CAD build for the part. Positions are in the model's coordinates, mm. A direction names the side the tool comes from. Round coordinates to 2 decimals unless told otherwise and drop trailing zeros. Write each loop counter-clockwise with the first axis right and the second up, starting at its lowest first coordinate (ties: lowest second). Pieces come first, ordered by that corner, then holes. Notation, with made-up numbers: (10, 32) -> (47, 32) arc R22 ccw to (47, 39) -> close; hole circle Ø8 at (80, 18.5). An arc over 180 degrees is marked (long way). Put each result on its own line as item: value. Start each with the question number.
1. Saw through at D-D on y = -9.25. List the corners of the cut face in (x, z), and give its area (3 significant figures).
2. Pull direction X, two halves, no side cores. Call faces 4 (the cylindrical face through (-7.908, -2.465, 5.805)), 5 (the flat face through (7, -5, -7)), 6 (the flat face through (0, -15, 0)), 7 (the cylindrical face through (-0.867, 0.296, -3.905)): pulls with the +X half, pulls with the -X half, needs draft (parallel to the pull), parting line crosses it, or undercut.
3. 3-axis set-ups, long thin cutter, end or side, ignore diameter. For faces 1 (the flat face through (-4, -10, 4)), 2 (the cylindrical face through (9.139, -7.395, 14.334)), 3 (the flat face through (6, -5, 6)): which of +Z, -Z, +X, -X, +Y, -Y reach the whole face in a straight line?
4. Saw through at B-B on x = 0. List the corners of the cut face in (y, z) (3 decimals).
5. Flat gauge pins, fed straight in: P1, Ø3, axis at x = -1.5, z = -5, coming from the +Y side; P2, Ø2.5, axis at x = 5.66, z = 5.66, coming from the +Y side; P3, Ø3, axis at y = -9.5, z = 6, coming from the -X side. Where does each tip first touch, or does it go through?
6. Saw through at A-A on y = -13. List the corners of the cut face in (x, z).
7. Saw through at C-C on z = 0. List the corners of the cut face in (x, y) (3 decimals), and give its area (3 significant figures).
8. Drill centre lines: line 1 (Z direction, x = -6, y = -4.5); line 2 (Y direction, x = -0.5, z = -6.5); line 3 (Y direction, x = 2, z = -3). Where is each one in solid material? Low to high. Write a range as from..to.
from build123d import *

# Parameters (mm, degrees)
F0_R     = 17
F0_R_2   = 1.5
F0_R_3   = 1
F0_R_4   = 4
F0_R_5   = 1.475
F1_DEPTH = 15
F2_START = 10
F2_DEPTH = 15
F3_DEPTH = 5
F4_DEPTH = 0.6
F5_DEPTH = 1.2


# Not quite as in the source:
# - a feature names something its author has since deleted; it is built from what else it names


with BuildPart() as f1:
    # F0 (on Front) → F1 (new body)
    with BuildSketch(Plane.XZ):
        Circle(F0_R)
        with BuildLine():
            ThreePointArc((-4.2152867015, -5.2422664968), (-4.1715341961, -5.447511614), (-4.1568542495, -5.6568542495))
            ThreePointArc((-4.1568542495, -5.6568542495), (-6.8551617286, -6.5591065343), (-5.2422664968, -4.2152867015))
            ThreePointArc((-5.2422664968, -4.2152867015), (-4.2289624147, -3.2427342391), (-3.2426406871, -4.2426406871))
            ThreePointArc((-3.2426406871, -4.2426406871), (-3.525928058, -4.9400093179), (-4.2152867015, -5.2422664968))
        make_face(mode=Mode.SUBTRACT)
        with Locations((6.7175144213, -6.7175144213)):
            Circle(F0_R_2, mode=Mode.SUBTRACT)
        with Locations((4.2426406871, -4.2426406871)):
            Circle(F0_R_3, mode=Mode.SUBTRACT)
        with Locations((-4.2426406871, 4.2426406871)):
            Circle(F0_R_3, mode=Mode.SUBTRACT)
        with Locations((-6.7175144213, 6.7175144213)):
            Circle(F0_R_2, mode=Mode.SUBTRACT)
        Circle(F0_R_4, mode=Mode.SUBTRACT)
        with BuildLine():
            ThreePointArc((4.2152867015, 5.2422664968), (5.447511614, 7.1421743029), (7.1568542495, 5.6568542495))
            ThreePointArc((7.1568542495, 5.6568542495), (6.5591065343, 4.4585467704), (5.2422664968, 4.2152867015))
            ThreePointArc((5.2422664968, 4.2152867015), (3.5355339059, 3.5355339059), (4.2152867015, 5.2422664968))
        make_face(mode=Mode.SUBTRACT)
        with BuildLine():
            ThreePointArc((5.2422664968, 4.2152867015), (6.5591065343, 4.4585467704), (7.1568542495, 5.6568542495))
            ThreePointArc((7.1568542495, 5.6568542495), (5.447511614, 7.1421743029), (4.2152867015, 5.2422664968))
            ThreePointArc((4.2152867015, 5.2422664968), (4.9400093179, 4.9593533163), (5.2426406871, 4.2426406871))
            ThreePointArc((5.2426406871, 4.2426406871), (5.2425471352, 4.2289624147), (5.2422664968, 4.2152867015))
        make_face()
        with BuildLine():
            ThreePointArc((5.2422664968, 4.2152867015), (4.5961940777, 4.5961940777), (4.2152867015, 5.2422664968))
            ThreePointArc((4.2152867015, 5.2422664968), (3.5355339059, 3.5355339059), (5.2422664968, 4.2152867015))
        make_face()
        with BuildLine():
            ThreePointArc((-5.2422664968, -4.2152867015), (-6.8551617286, -6.5591065343), (-4.1568542495, -5.6568542495))
            ThreePointArc((-4.1568542495, -5.6568542495), (-4.1715341961, -5.447511614), (-4.2152867015, -5.2422664968))
            ThreePointArc((-4.2152867015, -5.2422664968), (-4.9497474683, -4.9497474683), (-5.2422664968, -4.2152867015))
        make_face()
        with BuildLine():
            ThreePointArc((-5.2422664968, -4.2152867015), (-4.9497474683, -4.9497474683), (-4.2152867015, -5.2422664968))
            ThreePointArc((-4.2152867015, -5.2422664968), (-4.5961940777, -4.5961940777), (-5.2422664968, -4.2152867015))
        make_face()
        with BuildLine():
            ThreePointArc((-5.2422664968, -4.2152867015), (-4.5961940777, -4.5961940777), (-4.2152867015, -5.2422664968))
            ThreePointArc((-4.2152867015, -5.2422664968), (-3.525928058, -4.9400093179), (-3.2426406871, -4.2426406871))
            ThreePointArc((-3.2426406871, -4.2426406871), (-4.2289624147, -3.2427342391), (-5.2422664968, -4.2152867015))
        make_face()
        with BuildLine():
            ThreePointArc((5.2426406871, 4.2426406871), (4.9400093179, 4.9593533163), (4.2152867015, 5.2422664968))
            ThreePointArc((4.2152867015, 5.2422664968), (4.5961940777, 4.5961940777), (5.2422664968, 4.2152867015))
            ThreePointArc((5.2422664968, 4.2152867015), (5.2425471352, 4.2289624147), (5.2426406871, 4.2426406871))
        make_face()
        with Locations((4.2426406871, -4.2426406871)):
            Circle(F0_R_3)
        with Locations((-4.2426406871, 4.2426406871)):
            Circle(F0_R_3)
        with Locations((-6.7175144213, 6.7175144213)):
            Circle(F0_R_2)
        with Locations((6.7175144213, -6.7175144213)):
            Circle(F0_R_2)
        Circle(F0_R_4)
        Circle(F0_R_5, mode=Mode.SUBTRACT)
        Circle(F0_R_5)
    extrude(amount=F1_DEPTH)

    # F0 (on Front) → F2 (cut)
    with BuildSketch(Plane.XZ.offset(F2_START)):
        with BuildLine():
            ThreePointArc((-5.2422664968, -4.2152867015), (-4.5961940777, -4.5961940777), (-4.2152867015, -5.2422664968))
            ThreePointArc((-4.2152867015, -5.2422664968), (-3.525928058, -4.9400093179), (-3.2426406871, -4.2426406871))
            ThreePointArc((-3.2426406871, -4.2426406871), (-4.2289624147, -3.2427342391), (-5.2422664968, -4.2152867015))
        make_face()
        with BuildLine():
            ThreePointArc((-5.2422664968, -4.2152867015), (-4.9497474683, -4.9497474683), (-4.2152867015, -5.2422664968))
            ThreePointArc((-4.2152867015, -5.2422664968), (-4.5961940777, -4.5961940777), (-5.2422664968, -4.2152867015))
        make_face()
        with Locations((4.2426406871, -4.2426406871)):
            Circle(F0_R_3)
        with BuildLine():
            ThreePointArc((5.2422664968, 4.2152867015), (4.5961940777, 4.5961940777), (4.2152867015, 5.2422664968))
            ThreePointArc((4.2152867015, 5.2422664968), (3.5355339059, 3.5355339059), (5.2422664968, 4.2152867015))
        make_face()
        with BuildLine():
            ThreePointArc((5.2426406871, 4.2426406871), (4.9400093179, 4.9593533163), (4.2152867015, 5.2422664968))
            ThreePointArc((4.2152867015, 5.2422664968), (4.5961940777, 4.5961940777), (5.2422664968, 4.2152867015))
            ThreePointArc((5.2422664968, 4.2152867015), (5.2425471352, 4.2289624147), (5.2426406871, 4.2426406871))
        make_face()
        with Locations((-4.2426406871, 4.2426406871)):
            Circle(F0_R_3)
    extrude(amount=F2_DEPTH, mode=Mode.SUBTRACT)

    # F0 (on Front) → F3 (cut)
    with BuildSketch(Plane.XZ):
        with BuildLine():
            ThreePointArc((5.2422664968, 4.2152867015), (6.5591065343, 4.4585467704), (7.1568542495, 5.6568542495))
            ThreePointArc((7.1568542495, 5.6568542495), (5.447511614, 7.1421743029), (4.2152867015, 5.2422664968))
            ThreePointArc((4.2152867015, 5.2422664968), (4.9400093179, 4.9593533163), (5.2426406871, 4.2426406871))
            ThreePointArc((5.2426406871, 4.2426406871), (5.2425471352, 4.2289624147), (5.2422664968, 4.2152867015))
        make_face()
        with BuildLine():
            ThreePointArc((5.2426406871, 4.2426406871), (4.9400093179, 4.9593533163), (4.2152867015, 5.2422664968))
            ThreePointArc((4.2152867015, 5.2422664968), (4.5961940777, 4.5961940777), (5.2422664968, 4.2152867015))
            ThreePointArc((5.2422664968, 4.2152867015), (5.2425471352, 4.2289624147), (5.2426406871, 4.2426406871))
        make_face()
        with BuildLine():
            ThreePointArc((-5.2422664968, -4.2152867015), (-6.8551617286, -6.5591065343), (-4.1568542495, -5.6568542495))
            ThreePointArc((-4.1568542495, -5.6568542495), (-4.1715341961, -5.447511614), (-4.2152867015, -5.2422664968))
            ThreePointArc((-4.2152867015, -5.2422664968), (-4.9497474683, -4.9497474683), (-5.2422664968, -4.2152867015))
        make_face()
        with BuildLine():
            ThreePointArc((-5.2422664968, -4.2152867015), (-4.9497474683, -4.9497474683), (-4.2152867015, -5.2422664968))
            ThreePointArc((-4.2152867015, -5.2422664968), (-4.5961940777, -4.5961940777), (-5.2422664968, -4.2152867015))
        make_face()
        with Locations((6.7175144213, -6.7175144213)):
            Circle(F0_R_2)
        with Locations((-6.7175144213, 6.7175144213)):
            Circle(F0_R_2)
    extrude(amount=F3_DEPTH, mode=Mode.SUBTRACT)

    # F0 (on Front) → F4 (join)
    with BuildSketch(Plane.XZ):
        Circle(F0_R_4)
        Circle(F0_R_5, mode=Mode.SUBTRACT)
    extrude(amount=-F4_DEPTH)

    # F0 (on Front) → F5 (join)
    with BuildSketch(Plane.XZ):
        Circle(F0_R_5)
    extrude(amount=-F5_DEPTH)


solid = f1.part
Return value:
1. outline: circle Ø34 at (0, 0)
1. area: 908 mm^2
2. face 4: undercut
2. face 5: undercut
2. face 6: needs draft
2. face 7: parting line crosses it
3. face 1: -Y
3. face 2: +Y, -Y
3. face 3: +Y
4. outline: (-15, -17) -> (0, -17) -> (0, -4) -> (0.6, -4) -> (0.6, -1.475) -> (1.2, -1.475) -> (1.2, 1.475) -> (0.6, 1.475) -> (0.6, 4) -> (0, 4) -> (0, 17) -> (-15, 17) -> close
5. P1: stops at y = 0.6
5. P2: stops at y = -5
5. P3: stops at x = -16.39
6. outline: circle Ø34 at (0, 0); hole circle Ø2 at (-4.24, -4.24); hole circle Ø2 at (-4.24, 4.24); hole circle Ø2 at (4.24, -4.24); hole circle Ø2 at (4.24, 4.24)
7. outline: (-17, -15) -> (17, -15) -> (17, 0) -> (4, 0) -> (4, 0.6) -> (1.475, 0.6) -> (1.475, 1.2) -> (-1.475, 1.2) -> (-1.475, 0.6) -> (-4, 0.6) -> (-4, 0) -> (-17, 0) -> close
7. area: 517 mm^2
8. line 1: z = -15.91..-7.12, -4.2..5.4, 8.03..15.91
8. line 2: y = -15..0
8. line 3: y = -15..0.6
